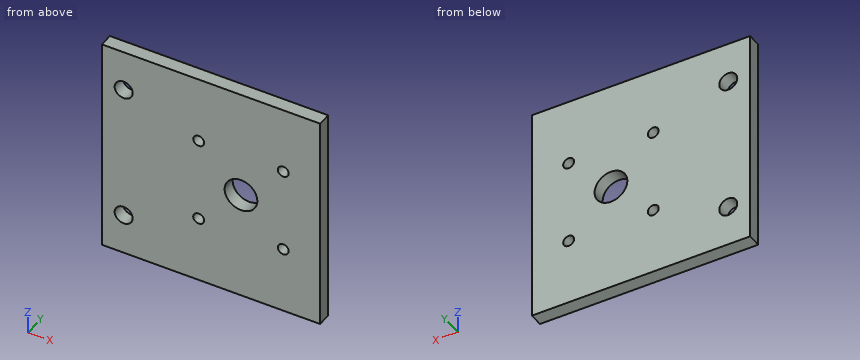
from build123d import *

# Parameters (mm, degrees)
SCHIZZO1_W                   = 80
SCHIZZO1_H                   = 5
ESTRUSIONE_ESTRUSIONE1_DEPTH = 80
FORO_PER_VITE_M6_1_D         = 6.6
SCHIZZO4_R                   = 6
TAGLIO_ESTRUSIONE1_DEPTH     = 114.247516529
SCHIZZO6_R                   = 2
TAGLIO_ESTRUSIONE3_DEPTH     = 114.247516529


with BuildPart() as part:
    # Schizzo1 → Estrusione-Estrusione1 (new body)
    with BuildSketch(Plane.XY):
        with Locations((40, 2.5)):
            Rectangle(SCHIZZO1_W, SCHIZZO1_H)
    extrude(amount=ESTRUSIONE_ESTRUSIONE1_DEPTH)

    # Foro per Vite M6-1 (through all)
    with Locations(Plane(origin=(0, 5, 0), x_dir=(1, 0, 0), z_dir=(0, 1, 0))):
        with Locations((8, -15), (8, -65)):
            Hole(FORO_PER_VITE_M6_1_D / 2)

    # Schizzo4 → Taglio-Estrusione1 (cut, through all)
    with BuildSketch(Plane(origin=(0, 5, 0), x_dir=(1, 0, 0), z_dir=(0, 1, 0))):
        with Locations(Location((51, -40, 0), (0, 0, 270))):
            Circle(SCHIZZO4_R)
    extrude(amount=-TAGLIO_ESTRUSIONE1_DEPTH, mode=Mode.SUBTRACT)

    # Schizzo6 → Taglio-Estrusione3 (cut, through all)
    with BuildSketch(Plane(origin=(0, 5, 0), x_dir=(1, 0, 0), z_dir=(0, 1, 0))):
        with Locations(Location((35.5, -24.5, 0), (0, 0, 270))):
            Circle(SCHIZZO6_R)
        with Locations(Location((66.5, -24.5, 0), (0, 0, 270))):
            Circle(SCHIZZO6_R)
        with Locations(Location((66.5, -55.5, 0), (0, 0, 270))):
            Circle(SCHIZZO6_R)
        with Locations(Location((35.5, -55.5, 0), (0, 0, 270))):
            Circle(SCHIZZO6_R)
    extrude(amount=-TAGLIO_ESTRUSIONE3_DEPTH, mode=Mode.SUBTRACT)


solid = part.part
Geometry: final body of the model. Coordinates: model frame, mm. Coordinates: 2 decimals unless noted, no trailing zeros. Order: outer loops, then holes, each group sorted by start corner. A loop starts at its lowest first (then second) coordinate and runs counter-clockwise, first axis right, second up. Notation, with made-up numbers: (32.5, -2) - (62.5, -2) arc R12 cw to (62.5, 6) - close; hole circle Ø2 at (3.25, 74.25). An arc over 180 degrees is marked (long way). Use one line per item in the form item = value.
1) Section B-B (x = 51). Return loops of the section in (y, z).
Solutions:
outline = (0, 0) - (5, 0) - (5, 34) - (0, 34) - close; (0, 46) - (5, 46) - (5, 80) - (0, 80) - close
2) Ray query, L1, parallel to X at y = 2, z = 55.5; L2, parallel to Z at x = 8, y = 1.15; L3, parallel to X at y = 0.75, z = 65. Return the intervals inside material, ascending.
Solutions:
L1 = 0 to 33.5, 37.5 to 64.5, 68.5 to 80
L2 = 0 to 11.7, 18.3 to 61.7, 68.3 to 80
L3 = 0 to 4.7, 11.3 to 80
3) Section D-D (y = 3.95). Return loops of the section in (x, z), then the cut area to 3 significant figures.
Solutions:
outline = (0, 0) - (80, 0) - (80, 80) - (0, 80) - close; hole circle Ø6.6 at (8, 15); hole circle Ø6.6 at (8, 65); hole circle Ø4 at (35.5, 24.5); hole circle Ø4 at (35.5, 55.5); hole circle Ø12 at (51, 40); hole circle Ø4 at (66.5, 24.5); hole circle Ø4 at (66.5, 55.5)
area = 6,170 mm^2
4) Section C-C (z = 24.5). Return loops of the section in (x, y), then the cut area to 3 significant figures.
Solutions:
outline = (0, 0) - (33.5, 0) - (33.5, 5) - (0, 5) - close; (37.5, 0) - (64.5, 0) - (64.5, 5) - (37.5, 5) - close; (68.5, 0) - (80, 0) - (80, 5) - (68.5, 5) - close
area = 360 mm^2
5) Section A-A (z = 40). Return loops of the section in (x, y), then the cut area to 3 significant figures.
Solutions:
outline = (0, 0) - (45, 0) - (45, 5) - (0, 5) - close; (57, 0) - (80, 0) - (80, 5) - (57, 5) - close
area = 340 mm^2
